Could you check a few things on this model? Use its own coordinates, in mm. Face numbers are marked on the shaded views. A direction names the side the tool comes from. Coordinates: 2 decimals unless noted, no trailing zeros. Order: outer loops, then holes, each group sorted by start corner. A loop starts at its lowest first (then second) coordinate and runs counter-clockwise, first axis right, second up. Notation, with made-up numbers: (60, -22.5) - (77, -22.5) arc R12 cw to (77, -13.5) - close; hole circle Ø3 at (53, 68.5). An arc over 180 degrees is marked (long way). Answer as a JSON object with one key per item and string values. Group by question number.
(1) Imagine slicing it at B-B, the plane x = 16.2. Write out the boundary of the cut face in (y, z), and give its area (3 significant figures).
(2) Imagine slicing it at D-D, the plane y = -8.2. Write out the boundary of the cut face in (x, z), and give its area (3 significant figures).
(3) We'd pull the mould along X, two halves only. Please class the marked faces 3, 4 and 5: pulls with the +X half, pulls with the -X half, needs draft (parallel to the pull), parting line crosses it, or undercut.
(4) Which directions (+Z, -Z, +X, -X, +Y, -Y) give clear straight access to the entire face, cutting with the end or side of a thin tool? Please do the marked faces 1 and 2.
(5) Will these pins go through, and if not, where does the flat tip stop? P1, Ø9.5, axis at x = -16.2, y = -8.2, coming from the -Z side; P2, Ø12, axis at x = 8, y = 0, coming from the +Z side; P3, Ø3, axis at x = 15.5, y = -7, coming from the -Z side.
(6) Imagine slicing it at A-A, the plane y = 8.2. Write out the boundary of the cut face in (x, z).
(7) Imagine slicing it at C-C, the plane z = 0.7. Write out the boundary of the cut face in (x, y), and give its area (3 significant figures).
(8) Please list where these lines run through material, in increasing order: probe 1 along Y at (x, z) = (-16.2, 1.5); probe 2 along Y at (x, z) = (16.2, 3.1); probe 3 along X at (y, z) = (-8.2, 0.7).
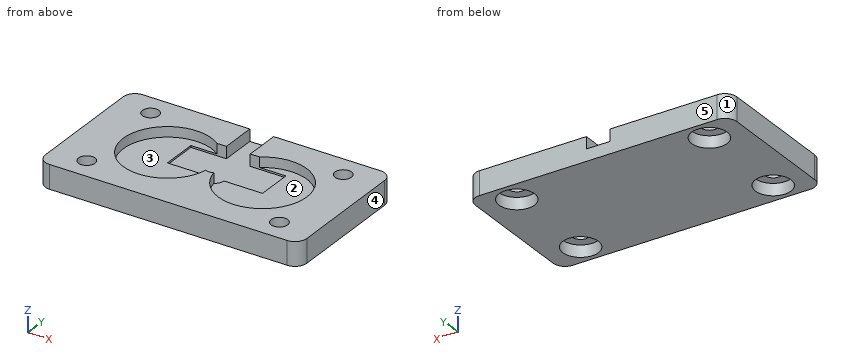
from build123d import *

# Parameters (mm, degrees)
SKETCH051_W         = 44
SKETCH051_H         = 24
PAD014_DEPTH        = 4
SKETCH052_R         = 7.45
POCKET015_DEPTH     = 1.7
SKETCH053_R         = 1.5
SKETCH053_W         = 16
SKETCH053_H         = 6
SKETCH053_W_2       = 4
POCKET016_DEPTH     = 2
HOLE022_D           = 2.8
HOLE022_DEPTH       = 25
HOLE022_CBORE_D     = 6
HOLE022_CBORE_DEPTH = 2
FILLET020_R         = 2


with BuildPart() as part:
    # Sketch051 → Pad014 (new body)
    with BuildSketch(Plane.XY):
        Rectangle(SKETCH051_W, SKETCH051_H)
    extrude(amount=PAD014_DEPTH)

    # Sketch052 (on Face6 of Pad014) → Pocket015 (cut)
    with BuildSketch(Plane.XY.offset(4)):
        with Locations((8, 0)):
            Circle(SKETCH052_R)
    pocket015 = extrude(amount=-POCKET015_DEPTH, mode=Mode.SUBTRACT)

    # Mirrored025: Pocket015 across Sketch052 V_Axis
    add(pocket015.mirror(Plane(origin=(0, 0, 4), x_dir=(0, 0, 1), z_dir=(1, 0, 0))), mode=Mode.SUBTRACT)

    # Sketch053 (on Face5 of Mirrored025) → Pocket016 (cut)
    with BuildSketch(Plane.XY.offset(4)):
        Circle(SKETCH053_R)
        with Locations((0, 3)):
            Rectangle(SKETCH053_W, SKETCH053_H)
        with Locations((0, 9)):
            Rectangle(SKETCH053_W_2, SKETCH053_H)
    extrude(amount=-POCKET016_DEPTH, mode=Mode.SUBTRACT)

    # Hole022
    with Locations(Plane(origin=(0, 0, 0), x_dir=(1, 0, 0), z_dir=(0, 0, -1))):
        with Locations((16.2, 8.2), (16.2, -8.2)):
            hole022 = CounterBoreHole(HOLE022_D / 2, HOLE022_CBORE_D / 2, HOLE022_CBORE_DEPTH, depth=HOLE022_DEPTH)

    # Mirrored026: Hole022 across Sketch054 V_Axis
    add(hole022.mirror(Plane(origin=(0, 0, 0), x_dir=(0, 0, -1), z_dir=(1, 0, 0))), mode=Mode.SUBTRACT)

    # Fillet020
    fillet020_edges = [part.edges().sort_by_distance(p)[0] for p in [
        (-22, 12, 2),
        (-22, -12, 2),
        (22, -12, 2),
        (22, 12, 2),
    ]]
    fillet(fillet020_edges, radius=FILLET020_R)


solid = part.part
Result set:
{
 "1": {"outline": "(-12, 0) - (-11.2, 0) - (-11.2, 2) - (-9.6, 2) - (-9.6, 4) - (-12, 4) - close; (-6.8, 2) - (-5.2, 2) - (-5.2, 0) - (5.2, 0) - (5.2, 2) - (6.8, 2) - (6.8, 4) - (-6.8, 4) - close; (9.6, 2) - (11.2, 2) - (11.2, 0) - (12, 0) - (12, 4) - (9.6, 4) - close", "area": "60.8 mm^2"},
 "2": {"outline": "(-22, 0) - (-19.2, 0) - (-19.2, 2) - (-17.6, 2) - (-17.6, 4) - (-22, 4) - close; (-14.8, 2) - (-13.2, 2) - (-13.2, 0) - (13.2, 0) - (13.2, 2) - (14.8, 2) - (14.8, 4) - (-14.8, 4) - close; (17.6, 2) - (19.2, 2) - (19.2, 0) - (22, 0) - (22, 4) - (17.6, 4) - close", "area": "141 mm^2"},
 "3": {"face 3": "undercut", "face 4": "pulls with the +X half", "face 5": "needs draft"},
 "4": {"face 1": "+Z, -Z, -X, +Y", "face 2": "+Z"},
 "5": {"P1": "stops at z = 0", "P2": "stops at z = 2.3", "P3": "stops at z = 2"},
 "6": {"outline": "(-22, 0) - (-19.2, 0) - (-19.2, 2) - (-17.6, 2) - (-17.6, 4) - (-22, 4) - close; (-14.8, 2) - (-13.2, 2) - (-13.2, 0) - (13.2, 0) - (13.2, 2) - (14.8, 2) - (14.8, 4) - (2, 4) - (2, 2) - (-2, 2) - (-2, 4) - (-14.8, 4) - close; (17.6, 2) - (19.2, 2) - (19.2, 0) - (22, 0) - (22, 4) - (17.6, 4) - close"},
 "7": {"outline": "(-22, -10) arc R2 ccw to (-20, -12) - (20, -12) arc R2 ccw to (22, -10) - (22, 10) arc R2 ccw to (20, 12) - (-20, 12) arc R2 ccw to (-22, 10) - close; hole circle Ø6 at (-16.2, -8.2); hole circle Ø6 at (-16.2, 8.2); hole circle Ø6 at (16.2, -8.2); hole circle Ø6 at (16.2, 8.2)", "area": "939 mm^2"},
 "8": {"probe 1": "y = -12 to -11.2, -5.2 to 5.2, 11.2 to 12", "probe 2": "y = -12 to -9.6, -6.8 to 6.8, 9.6 to 12", "probe 3": "x = -22 to -19.2, -13.2 to 13.2, 19.2 to 22"}
}
